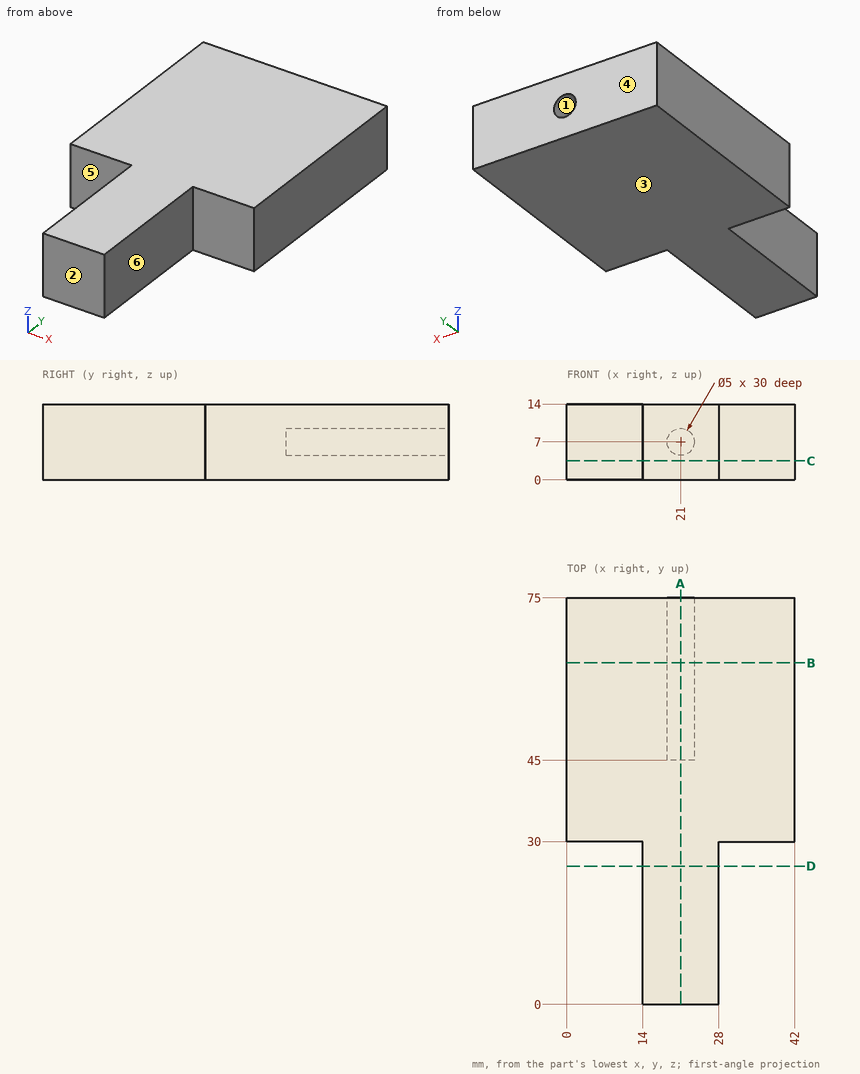
Geometry check sheet. Reference: drawing and pictorial views, mm from the part's lowest x, y, z. A direction names the side the tool comes from. Round coordinates to 2 decimals unless told otherwise and drop trailing zeros. Loops run counter-clockwise (first coordinate to the right, second up) from the corner with the lowest first, then second, coordinate; pieces in that order, holes last. Notation, with made-up numbers: M -40,8 L 19,8 A31 cw 19,41 Z; hole C 1.25,56.5 d8. An arc over 180 degrees is marked long. One line per item, written item: value.
(1) Sectioned sample at A-A, the plane x = 21. Record the cut outline in (y, z).
Computed values:
outline: M 0,0 L 75,0 L 75,4.5 L 45,4.5 L 45,9.5 L 75,9.5 L 75,14 L 0,14 Z
(2) Sectioned sample at B-B, the plane y = 63. Record the cut outline in (x, z), then the cut area to 3 significant figures.
Computed values:
outline: M 0,0 L 42,0 L 42,14 L 0,14 Z; hole C 21,7 d5
area: 568 mm^2
(3) Sectioned sample at D-D, the plane y = 25.5. Record the cut outline in (x, z), then the cut area to 3 significant figures.
Computed values:
outline: M 14,0 L 28,0 L 28,14 L 14,14 Z
area: 196 mm^2
(4) Thickness scan on line 1 (X direction, y = 56.25, z = 7); line 2 (Z direction, x = 21, y = 65); line 3 (X direction, y = 21.5, z = 10). Record the ranges inside material, lowest first.
Computed values:
line 1: x = 0 to 18.5, 23.5 to 42
line 2: z = 0 to 4.5, 9.5 to 14
line 3: x = 14 to 28
(5) Sectioned sample at C-C, the plane z = 3.5. Record the cut outline in (x, y), then the cut area to 3 significant figures.
Computed values:
outline: M 0,30 L 14,30 L 14,0 L 28,0 L 28,30 L 42,30 L 42,75 L 0,75 Z
area: 2,310 mm^2
(6) Release check for a two-part mould opening along Z. For the marked faces 1, 2 and 3 record: +Z half, -Z half, draft (parallel to the pull), parting line (faces both ways), or undercut.
Computed values:
face 1: undercut
face 2: draft
face 3: -Z half
(7) Depth check by flat-ended pin: pin 1 Ø7 at (y, z) = (18, 7.5) entering from +X; pin 2 Ø1 at (x, z) = (30, 6) entering from -Y. Enter the tip coordinate at first touch or a pass-through.
Computed values:
pin 1: stops at x = 28
pin 2: stops at y = 30
(8) Access from +Z, -Z, +X, -X, +Y, -Y to the whole of each face (thin tool, end or side, straight path). Record for the marked faces 4, 5 and 6.
Computed values:
face 4: +Z, -Z, +X, -X, +Y
face 5: +Z, -Z, -X, -Y
face 6: +Z, -Z, +X, -Y
